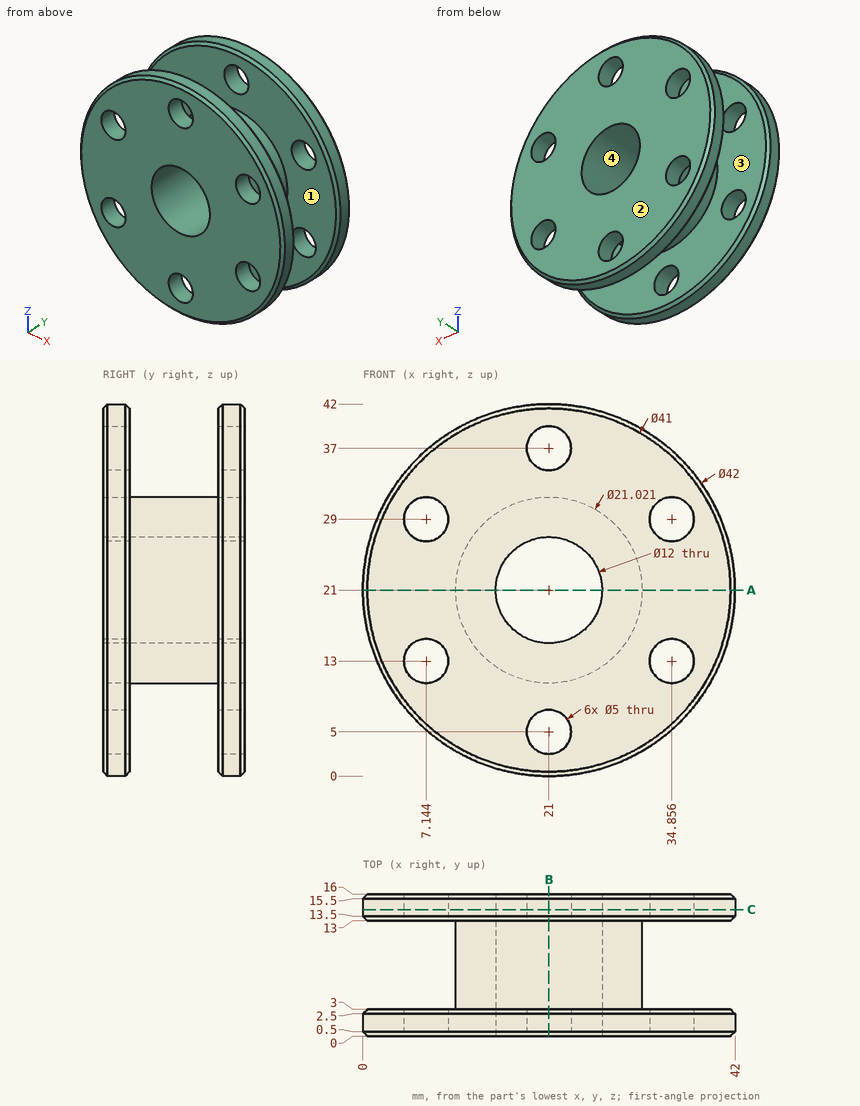
Here's the drawing with two shaded views (mm, measured from the low corner). I have some questions. A direction names the side the tool comes from. Give positions to 0.01 mm unless a question says otherwise; leave off trailing zeros. Order: outer loops, then holes, each group sorted by start corner. A loop starts at its lowest first (then second) coordinate and runs counter-clockwise, first axis right, second up.
Q1. For the marked faces 1 and 2, which set-ups out of +Z, -Z, +X, -X, +Y, -Y let a thin tool reach every point of the face, with its end or its side?
Q2. Suppose I cut it at A-A, the plane z = 21. Write out the boundary of the cut face in (x, y).
Q3. If I drill on line 1 along Y through (x, z) = (12.5, 39); line 2 along X through (y, z) = (1.6, 29) (1 decimal); line 3 along Z through (x, y) = (23, 10.75), over which ranges is the centre line in solid material (lowest first)?
Q4. Suppose I cut it at C-C, the plane y = 14.25. Write out the boundary of the cut face in (x, z).
Q5. We'd pull the mould along X, two halves only. Please class the marked faces 3 and 4: +X half, -X half, draft (parallel to the pull), parting line (faces both ways), or undercut.
Q6. Suppose I cut it at B-B, the plane x = 21. Count the separate pieces of the cut face and the enclosed holes in it, and give its area (3 significant figures).
Q7. I'm going to push flat-ended pins straight in: P1, Ø6, axis at y = 5.5, z = 13, coming from the -X side; P2, Ø4, axis at y = 4.5, z = 23.5, coming from the -X side (1 decimal); P3, Ø3, axis at y = 4, z = 11.5, coming from the -X side. Where does each tip first touch, or does it pass through?
Solution:
1. face 1: none
1. face 2: +Z, -Z, +X, -X, +Y
2. outline: (0, 0.5) - (0.5, 0) - (15, 0) - (15, 16) - (0.5, 16) - (0, 15.5) - (0, 13.5) - (0.5, 13) - (10.49, 13) - (10.49, 3) - (0.5, 3) - (0, 2.5) - close; (27, 0) - (41.5, 0) - (42, 0.5) - (42, 2.5) - (41.5, 3) - (31.51, 3) - (31.51, 13) - (41.5, 13) - (42, 13.5) - (42, 15.5) - (41.5, 16) - (27, 16) - close
3. line 1: y = 0 to 3, 13 to 16
3. line 2: x = 1.6 to 4.6, 9.6 to 32.4, 37.4 to 40.4
3. line 3: z = 10.68 to 15.34, 26.66 to 31.32
4. outline: circle Ø42 at (21, 21); hole circle Ø5 at (7.14, 13); hole circle Ø5 at (7.14, 29); hole circle Ø12 at (21, 21); hole circle Ø5 at (21, 5); hole circle Ø5 at (21, 37); hole circle Ø5 at (34.86, 13); hole circle Ø5 at (34.86, 29)
5. face 3: draft
5. face 4: undercut
6. separate pieces: 6
6. enclosed holes: 0
6. area: 209 mm2
7. P1: stops at x = 1.38
7. P2: stops at x = 0.1
7. P3: stops at x = 2.12
